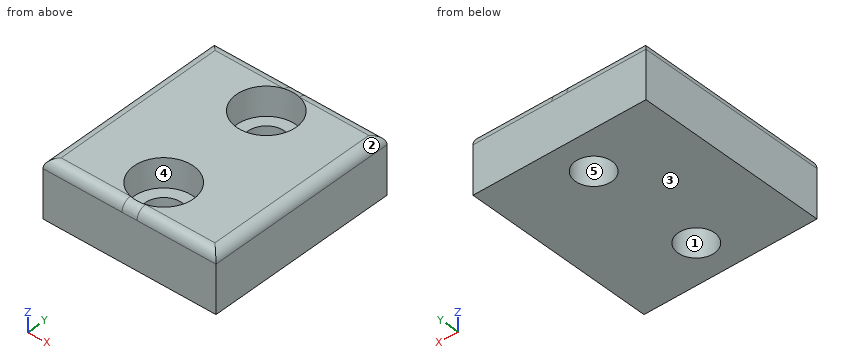
Autodesk Inventor part; units mm, degrees
ref_plane "YZ Plane" through (0, 0, 0) normal (1, 0, 0) x (0, 1, 0)
ref_plane "XZ Plane" through (0, 0, 0) normal (0, 1, 0) x (-1, 0, 0)
ref_plane "XY Plane" through (0, 0, 0) normal (0, 0, 1) x (1, 0, 0)
sketch "Sketch1" plane through (0, 0, 0) normal (0, 0, 1) x (1, 0, 0)
  line L0 (-9, 10) -> (9, 10)
  line L1 (9, 10) -> (9, -10)
  line L2 (9, -10) -> (-9, -10)
  line L3 (-9, -10) -> (-9, 10)
  line L4 (-9, 10) -> (9, -10) construction
  line L5 (9, 10) -> (-9, -10) construction
  line L6 (0, 0) -> (0, 6)
  line L7 (0, 0) -> (0, -6)
  circle A0 centre (0, 6) radius 1.9
  circle A1 centre (0, -6) radius 1.9
  dimension "d0" = 18
  dimension "d1" = 20
  dimension "d2" = 6
  dimension "d3" = 6
  dimension "d4" = 3.8
  dimension "d5" = 3.8
extrude "Extrusion1" add sketch "Sketch1" along normal blind 6
sketch "Sketch2" plane through (0, 0, 6) normal (0, 0, 1) x (1, 0, 0)
  circle A0 centre (0, 6) radius 1.9
  circle A1 centre (0, 6) radius 3.1
  circle A2 centre (0, -6) radius 1.9
  circle A3 centre (0, -6) radius 3.1
  point P0 (0, 0)
  dimension "d8" = 6.2
  dimension "d9" = 6.2
extrude "Extrusion2" cut sketch "Sketch2" against normal blind 3
fillet "Fillet1" radius 1 4 edges at (0, 10, 6) (-9, 0, 6) (0, -10, 6) (9, 0, 6)
properties part number "ChassisLegV1"
The listing builds one solid part. Answer for the finished solid, in the listing's coordinates (mm). Face numbers are marked on the shaded views. A direction names the side the tool comes from. Coordinates: 2 decimals unless noted, no trailing zeros. Loops run counter-clockwise (first coordinate to the right, second up) from the corner with the lowest first, then second, coordinate; pieces in that order, holes last. Notation, with made-up numbers: (-22.5, 42) -> (13.5, 42) arc R12 cw to (13.5, 59) -> close; hole circle Ø5 at (-20.75, 12). An arc over 180 degrees is marked (long way). Answer in a Markdown table with one row per item. Add a question column.
1. For the marked faces 4 and 5, determine the directions among +Z, -Z, +X, -X, +Y, -Y from which every point of the face is accessible in a straight line to the end or side of a thin tool.
2. The part is cut by section A-A, the plane y = 6. Write down the section's boundary in (x, z), then the cut area to 3 significant figures.
3. Flat-ended cylindrical pins translate along their axes: P1, Ø8, axis at x = 0, y = 6, coming from the -Z side; P2, Ø5.5, axis at x = 0, y = -6, coming from the +Z side. Find the tip coordinate at first contact, or state that the pin passes through.
4. Determine the mould class of the marked faces 1, 2 and 3 for opening direction X: +X half, -X half, draft (parallel to the pull), parting line (faces both ways), or undercut.
5. The part is cut by section B-B, the plane z = 2.25. Write down the section's boundary in (x, y), then the cut area to 3 significant figures.
6. The part is cut by section C-C, the plane x = 0. Count the separate pieces of the cut face and the enclosed holes in it, then the cut area to 3 significant figures.
7. Consider line 1 (Y direction, x = 0, z = 4.2); line 2 (X direction, y = -6, z = 4.8); line 3 (Y direction, x = 0, z = 1.2). Determine where each line is inside the solid, lowest interval first. Write a range as [from, to].
Answer below:
| question | item | result |
|---|---|---|
| 1 | face 4 | +Z |
| 1 | face 5 | +Z, -Z |
| 2 | outline | (-9, 0) -> (-1.9, 0) -> (-1.9, 3) -> (-3.1, 3) -> (-3.1, 6) -> (-8, 6) arc R1 ccw to (-9, 5) -> close; (1.9, 0) -> (9, 0) -> (9, 5) arc R1 ccw to (8, 6) -> (3.1, 6) -> (3.1, 3) -> (1.9, 3) -> close |
| 2 | area | 77.6 mm2 |
| 3 | P1 | z = 0 |
| 3 | P2 | z = 3 |
| 4 | face 1 | undercut |
| 4 | face 2 | +X half |
| 4 | face 3 | draft |
| 5 | outline | (-9, -10) -> (9, -10) -> (9, 10) -> (-9, 10) -> close; hole circle Ø3.8 at (0, -6); hole circle Ø3.8 at (0, 6) |
| 5 | area | 337 mm2 |
| 6 | separate pieces | 3 |
| 6 | enclosed holes | 0 |
| 6 | area | 59.6 mm2 |
| 7 | line 1 | [-10, -9.1], [-2.9, 2.9], [9.1, 10] |
| 7 | line 2 | [-9, -3.1], [3.1, 9] |
| 7 | line 3 | [-10, -7.9], [-4.1, 4.1], [7.9, 10] |
